```python
from build123d import *

# Parameters (mm, degrees)
BOSS_EXTRUDE1_DEPTH         = 12.7
BOSS_EXTRUDE1_DEPTH_BACK    = 12.7
SKETCH1_W                   = 76.2
SKETCH1_H                   = 203.2
SKETCH2_R                   = 4.7625
CUT_EXTRUDE1_DEPTH          = 25.4
CUT_EXTRUDE2_DEPTH          = 15.875
SKETCH5_W                   = 38.1
SKETCH5_H                   = 8.128
CUT_EXTRUDE4_DEPTH          = 110.249530891
F_1_4_20_TAPPED_HOLE1_D     = 5.1054
F_1_4_20_TAPPED_HOLE1_DEPTH = 19.05
F_1_4_20_TAPPED_HOLE1_TIP   = 1.533816902
SKETCH9_R                   = 2.5527
CUT_EXTRUDE5_DEPTH          = 112.44204772


with BuildPart() as part:
    # Sketch1 → Boss-Extrude1 (new, two sides: drawn at the far end of the back side and taken through both)
    with BuildSketch(Plane(origin=(0, 0, 0), x_dir=(1, 0, 0), z_dir=(0, 1, 0)).offset(-BOSS_EXTRUDE1_DEPTH_BACK)):
        Rectangle(SKETCH1_W, SKETCH1_H)
    extrude(amount=BOSS_EXTRUDE1_DEPTH + BOSS_EXTRUDE1_DEPTH_BACK)

    # Sketch2 → Cut-Extrude1 (cut)
    with BuildSketch(Plane(origin=(0, 0, -101.6), x_dir=(-1, 0, 0), z_dir=(0, 0, -1))):
        with Locations((0, -12.7)):
            Circle(SKETCH2_R)
    extrude(amount=-CUT_EXTRUDE1_DEPTH, mode=Mode.SUBTRACT)

    # Sketch3 → Cut-Extrude2 (cut)
    with BuildSketch(Plane(origin=(0, -12.7, 0), x_dir=(-1, 0, 0), z_dir=(0, -1, 0))):
        with BuildLine():
            Line((-19.05, -96.8375), (19.05, -96.8375))
            ThreePointArc((19.05, -96.8375), (23.540128061, -94.977628061), (25.4, -90.4875))
            Line((25.4, -90.4875), (25.4, 9.525))
            Line((25.4, 9.525), (44.45, 9.525))
            Line((44.45, 9.525), (44.45, 47.625))
            Line((44.45, 47.625), (-44.45, 47.625))
            Line((-44.45, 47.625), (-44.45, 9.525))
            Line((-44.45, 9.525), (-25.4, 9.525))
            Line((-25.4, 9.525), (-25.4, -90.4875))
            ThreePointArc((-25.4, -90.4875), (-23.540128061, -94.977628061), (-19.05, -96.8375))
        make_face()
        with BuildLine():
            Line((-22.225, 76.2), (22.225, 76.2))
            ThreePointArc((22.225, 76.2), (24.47006403, 75.27006403), (25.4, 73.025))
            Line((25.4, 73.025), (25.4, 71.247))
            ThreePointArc((25.4, 71.247), (24.47006403, 69.00193597), (22.225, 68.072))
            Line((22.225, 68.072), (-22.225, 68.072))
            ThreePointArc((-22.225, 68.072), (-24.47006403, 69.00193597), (-25.4, 71.247))
            Line((-25.4, 71.247), (-25.4, 73.025))
            ThreePointArc((-25.4, 73.025), (-24.47006403, 75.27006403), (-22.225, 76.2))
        make_face()
    extrude(amount=-CUT_EXTRUDE2_DEPTH, mode=Mode.SUBTRACT)

    # Sketch5 → Cut-Extrude4 (cut, through all)
    with BuildSketch(Plane(origin=(0, 0, 0), x_dir=(1, 0, 0), z_dir=(0, 1, 0))):
        with Locations((0, 72.136)):
            Rectangle(SKETCH5_W, SKETCH5_H)
    extrude(amount=CUT_EXTRUDE4_DEPTH, mode=Mode.SUBTRACT)

    # 1_4-20 Tapped Hole1
    with Locations(Plane(origin=(-11.034450397, 12.7, 14.547513529), x_dir=(-1, 0, 0), z_dir=(0, 1, 0))):
        with Locations((-11.034450397, -52.647513529)):
            Hole(F_1_4_20_TAPPED_HOLE1_D / 2, depth=F_1_4_20_TAPPED_HOLE1_DEPTH)
            with Locations((0, 0, -(F_1_4_20_TAPPED_HOLE1_DEPTH + F_1_4_20_TAPPED_HOLE1_TIP / 2))):  # 118° drill point
                Cone(0, F_1_4_20_TAPPED_HOLE1_D / 2, F_1_4_20_TAPPED_HOLE1_TIP, mode=Mode.SUBTRACT)

    # Sketch9 → Cut-Extrude5 (cut, through all)
    with BuildSketch(Plane(origin=(0, -12.7, 0), x_dir=(-1, 0, 0), z_dir=(0, -1, 0))):
        with Locations(Location((31.75, 57.15, 0), (0, 0, 90))):
            Circle(SKETCH9_R)
        with Locations(Location((31.75, 0, 0), (0, 0, 90))):
            Circle(SKETCH9_R)
        with Locations(Location((-31.75, 0, 0), (0, 0, 270))):
            Circle(SKETCH9_R)
        with Locations(Location((-31.75, 57.15, 0), (0, 0, 270))):
            Circle(SKETCH9_R)
    extrude(amount=-CUT_EXTRUDE5_DEPTH, mode=Mode.SUBTRACT)


solid = part.part
```
Here's how the part is built. I have some questions about the finished solid (model axes, mm). A direction names the side the tool comes from. Round coordinates to 2 decimals unless told otherwise and drop trailing zeros. Loops run counter-clockwise (first coordinate to the right, second up) from the corner with the lowest first, then second, coordinate; pieces in that order, holes last. Notation, with made-up numbers: (65.25, 18.5) -> (112.25, 18.5) arc R15 cw to (112.25, 43.5) -> close; hole circle Ø1 at (29, 15.5). An arc over 180 degrees is marked (long way). Answer as CSV lines item,"result". Start each with the question number.
1. Imagine slicing it at B-B on z = -38.1. Write out the boundary of the cut face in (x, y) (3 decimals), plus the area to 3 significant figures.
2. For faces 1 (the face through (-19.05, 8, -72)), 2 (the face through (-1, -5, -47.625)), 3 (the face through (25.4, -5, 40)), which set-ups out of +Z, -Z, +X, -X, +Y, -Y let a thin tool reach every point of the face, with its end or its side?
3. Imagine slicing it at C-C on x = 11. Write out the boundary of the cut face in (y, z) (1 decimal), plus the area to 3 significant figures.
4. If we mould it in two halves opening along X, with no side actions, what happens to faces 4 (the face through (-23.49, -4.874, 95.027)), 5 (the face through (32, -5, -9.525)), 6 (the face through (38.1, 0, 1)), 7 (the face through (-0.33, 7.87, -35.57))? For each: pulls with the +X half, pulls with the -X half, needs draft (parallel to the pull), parting line crosses it, or undercut.
5. I'm going to push a flat-ended pin straight in: P1, Ø1.9, axis at x = 22.5, z = -73, coming from the -Y side (3 decimals). Where does the tip first touch, or does it pass through?
6. Imagine slicing it at D-D on z = 0. Write out the boundary of the cut face in (x, y) (3 decimals), plus the area to 3 significant figures.
7. I need wall thicknesses on probe 1 along Z at (x, y) = (13.5, -1.25) (1 decimal); probe 2 along X at (y, z) = (-1.75, 0); probe 3 along Z at (x, y) = (31.75, 7.5). Which ranges of each line are inside material? Lowest first, please. Write a range as from..to.
8. Imagine slicing it at A-A on x = -31.75. Write out the boundary of the cut face in (y, z) (3 decimals).
Solution:
1,outline,"(-38.1, 3.175) -> (-2.553, 3.175) -> (-2.553, 12.7) -> (-38.1, 12.7) -> close; (2.553, 3.175) -> (38.1, 3.175) -> (38.1, 12.7) -> (2.553, 12.7) -> close"
1,area,"677 mm²"
2,face 1,"+Y, -Y"
2,face 2,"+X, -X, -Y"
2,face 3,"-Y"
3,outline,"(-12.7, -101.6) -> (12.7, -101.6) -> (12.7, -76.2) -> (-12.7, -76.2) -> close; (-12.7, -68.1) -> (12.7, -68.1) -> (12.7, 101.6) -> (-12.7, 101.6) -> (-12.7, 96.8) -> (3.2, 96.8) -> (3.2, -47.6) -> (-12.7, -47.6) -> close"
3,area,"2,660 mm²"
4,face 4,"undercut"
4,face 5,"needs draft"
4,face 6,"pulls with the +X half"
4,face 7,"undercut"
5,P1,"y = 3.175"
6,outline,"(-38.1, -12.7) -> (-34.303, -12.7) -> (-34.303, 12.7) -> (-38.1, 12.7) -> close; (-29.197, -12.7) -> (-25.4, -12.7) -> (-25.4, 3.175) -> (25.4, 3.175) -> (25.4, -12.7) -> (29.197, -12.7) -> (29.197, 12.7) -> (-29.197, 12.7) -> close; (34.303, -12.7) -> (38.1, -12.7) -> (38.1, 12.7) -> (34.303, 12.7) -> close"
6,area,"870 mm²"
7,probe 1,"-101.6..-76.2, -68.1..-47.6, 96.8..101.6"
7,probe 2,"-38.1..-34.3, -29.2..-25.4, 25.4..29.2, 34.3..38.1"
7,probe 3,"-101.6..-59.7, -54.6..-2.55, 2.55..101.6"
8,outline,"(-12.7, -101.6) -> (12.7, -101.6) -> (12.7, -59.703) -> (-12.7, -59.703) -> close; (-12.7, -54.597) -> (12.7, -54.597) -> (12.7, -2.553) -> (-12.7, -2.553) -> (-12.7, -9.525) -> (3.175, -9.525) -> (3.175, -47.625) -> (-12.7, -47.625) -> close; (-12.7, 2.553) -> (12.7, 2.553) -> (12.7, 101.6) -> (-12.7, 101.6) -> close"
